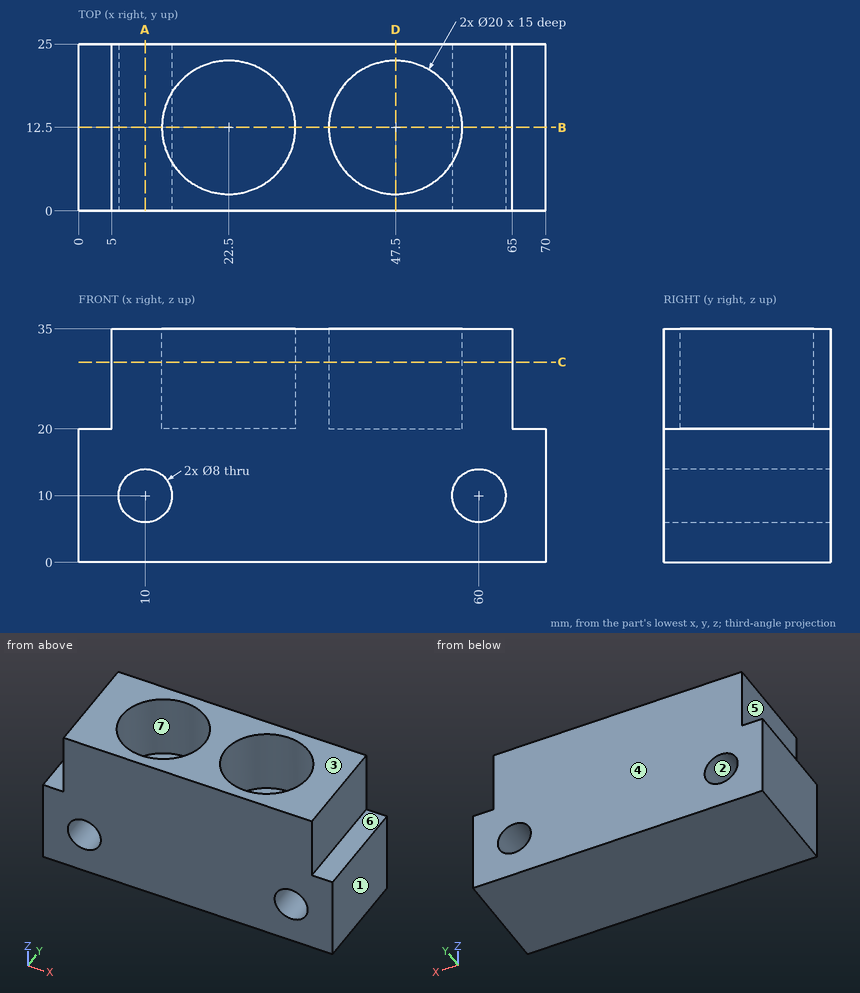
Part print with two shaded views. Sizes in mm from the minimum x, y, z corner. A direction names the side the tool comes from. Coordinates: 2 decimals unless noted, no trailing zeros. Order: outer loops, then holes, each group sorted by start corner. A loop starts at its lowest first (then second) coordinate and runs counter-clockwise, first axis right, second up. Notation, with made-up numbers: (24, 7.5) - (37, 7.5) arc R13 cw to (37, 29.5) - close; hole circle Ø9 at (-25.5, -37.75). An arc over 180 degrees is marked (long way). Answer in a Markdown table with one row per item.
1. Pull direction X, two halves, no side cores. Call the marked faces 1, 2 and 3: +X half, -X half, draft (parallel to the pull), parting line (faces both ways), or undercut.
Answer:
| item | result |
|---|---|
| face 1 | +X half |
| face 2 | undercut |
| face 3 | draft |
2. Flat gauge pins, fed straight in: P1, Ø6, axis at x = 26.5, y = 20.5, coming from the -Z side; P2, Ø2, axis at x = 8.5, z = 10, coming from the +Y side (3 decimals); P3, Ø5.5, axis at x = 68, y = 9, coming from the +Z side; P4, Ø4.5, axis at y = 9.5, z = 28, coming from the +X side. Where does each tip first touch, or does it go through?
Answer:
| item | result |
|---|---|
| P1 | z = 0 |
| P2 | through |
| P3 | z = 20 |
| P4 | x = 65 |
3. Drill centre lines: L1, parallel to Y at x = 47.5, z = 29.75; L2, parallel to X at y = 19, z = 23; L3, parallel to X at y = 6.25, z = 8.5. Where is each one in solid material? Low to high. Write a range as from..to.
Answer:
| item | result |
|---|---|
| L1 | 0..2.5, 22.5..25 |
| L2 | 5..14.9, 30.1..39.9, 55.1..65 |
| L3 | 0..6.29, 13.71..56.29, 63.71..70 |
4. Slice it at B-B, the plane y = 12.5. List the corners of the cut face in (x, z), then the cut area to 3 significant figures.
Answer:
| item | result |
|---|---|
| outline | (0, 0) - (70, 0) - (70, 20) - (65, 20) - (65, 35) - (57.5, 35) - (57.5, 20) - (37.5, 20) - (37.5, 35) - (32.5, 35) - (32.5, 20) - (12.5, 20) - (12.5, 35) - (5, 35) - (5, 20) - (0, 20) - close; hole circle Ø8 at (10, 10); hole circle Ø8 at (60, 10) |
| area | 1,600 mm² |
5. 3-axis set-ups, long thin cutter, end or side, ignore diameter. For the marked faces 4, 5, 6 and 7: which of +Z, -Z, +X, -X, +Y, -Y reach the whole face in a straight line?
Answer:
| item | result |
|---|---|
| face 4 | +Z, -Z, +X, -X, +Y |
| face 5 | +Z, -X, +Y, -Y |
| face 6 | +Z, +X, +Y, -Y |
| face 7 | +Z |
6. Slice it at A-A, the plane x = 10. List the corners of the cut face in (y, z), then the cut area to 3 significant figures.
Answer:
| item | result |
|---|---|
| outline | (0, 0) - (25, 0) - (25, 6) - (0, 6) - close; (0, 14) - (25, 14) - (25, 35) - (0, 35) - close |
| area | 675 mm² |
7. Slice it at D-D, the plane x = 47.5. List the corners of the cut face in (y, z), then the cut area to 3 significant figures.
Answer:
| item | result |
|---|---|
| outline | (0, 0) - (25, 0) - (25, 35) - (22.5, 35) - (22.5, 20) - (2.5, 20) - (2.5, 35) - (0, 35) - close |
| area | 575 mm² |
8. Slice it at C-C, the plane z = 30. List the corners of the cut face in (x, y), then the cut area to 3 significant figures.
Answer:
| item | result |
|---|---|
| outline | (5, 0) - (65, 0) - (65, 25) - (5, 25) - close; hole circle Ø20 at (22.5, 12.5); hole circle Ø20 at (47.5, 12.5) |
| area | 872 mm² |
